from build123d import *

# Parameters (mm, degrees)
F0_W     = 102.589286
F0_H     = 95.357146
F1_DEPTH = 25
F2_R     = 9.568015
F2_R_2   = 9.516545
F2_R_3   = 9.720787
F2_R_4   = 9.466873
F3_DEPTH = 25
F4_W     = 84.966198
F4_H     = 69.23151
F5_DEPTH = 30
F6_R     = 5


with BuildPart() as f1:
    # F0 (on Top) → F1 (new body)
    with BuildSketch(Plane.XY):
        with Locations((-1.875002, -0.13393)):
            Rectangle(F0_W, F0_H)
    extrude(amount=F1_DEPTH)

    # F2 (on face) → F3 (join)
    with BuildSketch(Plane.XY.offset(25)):
        with Locations((14.719443, 16.544643)):
            Circle(F2_R)
        with Locations((-18.169645, 16.544643)):
            Circle(F2_R_2)
        with Locations((-18.169645, -16.812503)):
            Circle(F2_R_3)
        with Locations((14.419641, -16.812503)):
            Circle(F2_R_4)
    extrude(amount=F3_DEPTH)

    # F4 (on face) → F5 (join)
    with BuildSketch(Plane.XY.offset(50)):
        Rectangle(F4_W, F4_H)
    extrude(amount=F5_DEPTH)

    # F6
    f6_edges = [f1.edges().sort_by_distance(p)[0] for p in [
        (42.483099, 0, 80),
        (0, -34.615755, 80),
        (-42.483099, 0, 80),
        (0, 34.615755, 80),
        (42.483099, -34.615755, 65),
        (42.483099, 34.615755, 65),
        (-42.483099, 34.615755, 65),
        (-42.483099, -34.615755, 65),
        (0, -34.615755, 50),
        (-42.483099, 0, 50),
        (0, 34.615755, 50),
        (42.483099, 0, 50),
    ]]
    fillet(f6_edges, radius=F6_R)


solid = f1.part
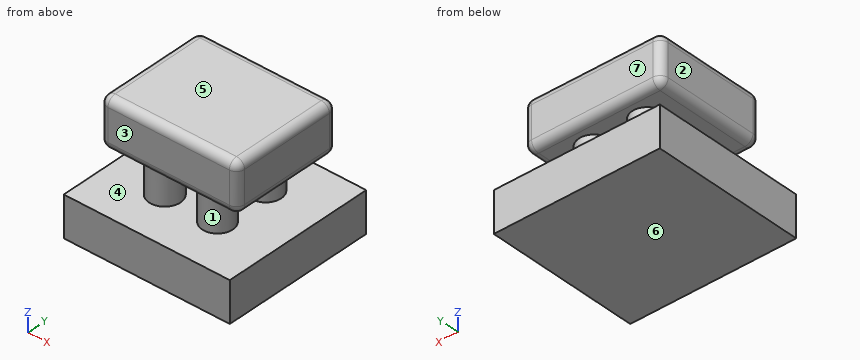
Part model, mm, in its own coordinate system. Face numbers are marked on the shaded views. A direction names the side the tool comes from. Give positions to 0.01 mm unless a question says otherwise; leave off trailing zeros. Loops run counter-clockwise (first coordinate to the right, second up) from the corner with the lowest first, then second, coordinate; pieces in that order, holes last.
(1) Band-saw the part on A-A (x = -35.5). Write the cut outline in (y, z), and give its area (3 significant figures).
Return value:
outline: (-47.81, 0) - (47.54, 0) - (47.54, 25) - (-47.81, 25) - close; (-34.62, 55) arc R5 ccw to (-29.62, 50) - (29.62, 50) arc R5 ccw to (34.62, 55) - (34.62, 75) arc R5 ccw to (29.62, 80) - (-29.62, 80) arc R5 ccw to (-34.62, 75) - close
area: 4,440 mm2
(2) Pin check, flat tips, straight feed: pin 1 (22 mm diameter, centred on x = -16.5, z = 60, fed in from +Y); pin 2 (6 mm diameter, centred on x = 8.5, z = 68.5, fed in from -Y); pin 3 (16 mm diameter, centred on y = 4, z = 66.5, fed in from +X); pin 4 (12 mm diameter, centred on x = 33, z = 32, fed in from -Y). Stop position of each tip, or through.
Return value:
pin 1: stops at y = 34.62
pin 2: stops at y = -34.62
pin 3: stops at x = 42.48
pin 4: passes through
(3) Band-saw the part on D-D (y = 18). Write the cut outline in (x, z), and give its area (3 significant figures).
Return value:
outline: (-53.17, 0) - (49.42, 0) - (49.42, 25) - (24.18, 25) - (24.18, 50) - (37.48, 50) arc R5 ccw to (42.48, 55) - (42.48, 75) arc R5 ccw to (37.48, 80) - (-37.48, 80) arc R5 ccw to (-42.48, 75) - (-42.48, 55) arc R5 ccw to (-37.48, 50) - (-27.57, 50) - (-27.57, 25) - (-53.17, 25) - close; hole (-8.77, 25) - (5.26, 25) - (5.26, 50) - (-8.77, 50) - close
area: 6,040 mm2
(4) Band-saw the part on B-B (z = 73). Write the cut outline in (x, y).
Return value:
outline: (-42.48, -29.62) arc R5 ccw to (-37.48, -34.62) - (37.48, -34.62) arc R5 ccw to (42.48, -29.62) - (42.48, 29.62) arc R5 ccw to (37.48, 34.62) - (-37.48, 34.62) arc R5 ccw to (-42.48, 29.62) - close
(5) Pull direction Z, two halves, no side cores. Call the marked faces 4, 5, 6 and 7: pulls with the +Z half, pulls with the -Z half, needs draft (parallel to the pull), parting line crosses it, or undercut.
Return value:
face 4: undercut
face 5: pulls with the +Z half
face 6: pulls with the -Z half
face 7: needs draft
(6) Drill centre lines: line 1 along Z through (x, y) = (19.5, 2.5); line 2 along Z through (x, y) = (-45, -37.5); line 3 along X through (y, z) = (2.5, 61). Where is each one in solid material? Low to high.
Return value:
line 1: z = 0 to 25, 50 to 80
line 2: z = 0 to 25
line 3: x = -42.48 to 42.48
(7) Band-saw the part on C-C (x = -11). Write the cut outline in (y, z).
Return value:
outline: (-47.81, 0) - (47.54, 0) - (47.54, 25) - (22.8, 25) - (22.8, 50) - (29.62, 50) arc R5 ccw to (34.62, 55) - (34.62, 75) arc R5 ccw to (29.62, 80) - (-29.62, 80) arc R5 ccw to (-34.62, 75) - (-34.62, 55) arc R5 ccw to (-29.62, 50) - (-23.38, 50) - (-23.38, 25) - (-47.81, 25) - close; hole (-10.25, 25) - (10.29, 25) - (10.29, 50) - (-10.25, 50) - close
(8) 3-axis set-ups, long thin cutter, end or side, ignore diameter. For the marked faces 1, 2 and 3: which of +Z, -Z, +X, -X, +Y, -Y reach the whole face in a straight line?
Return value:
face 1: none
face 2: +Z, -X, +Y, -Y
face 3: +Z, +X, -X, -Y
